Autodesk Inventor part; units mm, degrees
ref_plane "YZ Plane" through (0, 0, 0) normal (1, 0, 0) x (0, 1, 0)
ref_plane "XZ Plane" through (0, 0, 0) normal (0, 1, 0) x (-1, 0, 0)
ref_plane "XY Plane" through (0, 0, 0) normal (0, 0, 1) x (1, 0, 0)
sketch "Sketch1" plane through (0, 0, 0) normal (0, 0, 1) x (1, 0, 0)
  line L0 (-282.4704, -20.4341) -> (-282.4704, 20.4341)
  line L1 (-394.804, 0) -> (382.9893, 0) construction
  arc A0 (245.5307, -6.7859) -> (-282.4704, -20.4341) centre (0, -728.1449) ccw
  arc A1 (257.8072, 29.282) -> (-282.4704, 20.4341) centre (0, -728.1449) ccw
  line L2 (245.5307, -6.7859) -> (257.8072, 29.282)
  line L3 (257.8072, 29.282) -> (259.8533, 35.2933)
  line L4 (259.8533, 35.2933) -> (271.8759, 31.2011)
  line L5 (271.8759, 31.2011) -> (255.5072, -16.8895)
  line L6 (255.5072, -16.8895) -> (243.4846, -12.7973)
  line L7 (243.4846, -12.7973) -> (245.5307, -6.7859)
  line L8 (0, 237.1551) -> (0, -889.0282) construction
  line L9 (0, -728.1449) -> (-282.4704, 0) construction
  arc A2 (205.7125, -1.0346) -> (-280.1164, -26.3317) centre (0, -728.1449) ccw
  line L10 (-280.1164, -26.3317) -> (-282.4704, -20.4341)
  line L11 (243.4846, -12.7973) -> (245.5307, -6.7859)
  point P0 (0, 0)
  point P1 (205.7125, -1.0346)
  dimension "d65" = 762
  dimension "d67" = 50.8
  dimension "d68" = 38.1
  dimension "d69" = 12.7
  dimension "d76" = 40
  dimension "d97" = 800.1
  dimension "d98" = 6.35
extrude "Plate1" add sketch "Sketch1" along normal blind 4.7625 contours L0 A1 L2 A0
sketch "Sketch3" plane through (0, 0, 0) normal (0, 0, -1) x (-1, 0, 0)
  line L0 (269.2384, 95.4765) -> (282.4704, 20.4341)
  arc A0 (282.4704, 20.4341) -> (-257.8072, 29.282) centre (0, -728.1449) ccw
  arc A1 (282.4704, -20.4341) -> (-245.5307, -6.7859) centre (0, -728.1449) ccw construction
  line L1 (0, -900.8528) -> (0, 308.1027) construction
  line L2 (-366.2845, 0) -> (393.0567, 0) construction
  arc A2 (269.2384, 95.4765) -> (108.3857, 131.5609) centre (0, -728.1449) ccw
  arc A3 (108.3857, 131.5609) -> (104.0502, 97.172) centre (106.218, 114.3664) ccw
  arc A4 (203.8267, 78.347) -> (104.0502, 97.172) centre (0, -728.1449) ccw
  arc A5 (209.7927, 71.9287) -> (203.8267, 78.347) centre (201.8507, 70.5283) ccw
  line L3 (209.7927, 71.9287) -> (212.772, 55.032)
  arc A6 (202.7861, 45.8305) -> (212.772, 55.032) centre (204.8301, 53.6316) ccw
  point P0 (0, 0)
  point P1 (-2.2036, 71.9521)
  dimension "d70" = 80
  dimension "d88" = 165.1
  dimension "d91" = 76.2
  dimension "d92" = 101.6
  dimension "d93" = 8.0645
  dimension "d95" = 31.75
sheet face with bend "Face2" sketch "Sketch3" thickness 4.7625 toward (0, 0, 1) bend radius 4.7625
bend "Bend1"
sketch "Sketch5" plane through (0, 0, 0) normal (0, 0, -1) x (-1, 0, 0)
  arc A0 (282.4704, -20.4341) -> (-245.5307, -6.7859) centre (0, -728.1449) ccw construction
  spline S0 degree 3 poles (-4.2317, 35.5309) (-3.9947, 36.2065) (-3.5205, 37.5578) (-2.7876, 39.577) (-2.0409, 41.5912) (-1.5294, 42.9288) (-1.2737, 43.5976) knots 0 0 0 0 0.214807 0.429614 0.644422 0.859229 0.859229 0.859229 0.859229
  spline S1 degree 3 poles (4.2317, 35.5309) (3.9947, 36.2065) (3.5205, 37.5578) (2.7876, 39.577) (2.0409, 41.5912) (1.5294, 42.9288) (1.2737, 43.5976) knots 0 0 0 0 0.214807 0.429614 0.644422 0.859229 0.859229 0.859229 0.859229
  circle A1 centre (0, -728.1449) radius 763.6875
  arc A2 (1.2737, 43.5976) -> (-1.2737, 43.5976) centre (0, -728.1449) ccw
  point P0 (-3.5169, 37.5565)
  point P1 (-2.7853, 39.5762)
  point P2 (-2.0375, 41.5899)
  point P3 (3.5169, 37.5565)
  point P4 (2.7853, 39.5762)
  point P5 (2.0375, 41.5899)
extrude "Extrusion1" [suppressed]
pattern_circular "Circular Pattern1" [suppressed]
sketch "Sketch4" plane through (0, 0, 0) normal (0, 0, -1) x (-1, 0, 0)
  line L0 (282.4704, 20.4341) -> (269.2384, 95.4765) construction
  circle A0 centre (198.5568, 63.04) radius 25.4 construction
  line L1 (177.7503, 77.6089) -> (213.1256, 83.8465) construction
  line L2 (213.1256, 83.8465) -> (183.9879, 42.2336) construction
  line L3 (183.9879, 42.2336) -> (219.3632, 48.4712) construction
  line L4 (173.5426, 58.6294) -> (223.5709, 67.4507) construction
  line L5 (282.4704, 20.4341) -> (269.2384, 95.4765) construction
  line L6 (262.3523, 61.393) -> (265.6603, 42.6324) construction
  line L7 (0, -43.6162) -> (0, 118.6586) construction
  point P0 (0, 0)
  point P1 (257.9416, 86.4071)
  point P2 (272.2763, 5.1112)
  dimension "d31" = 25.4
  dimension "d33" = 12.7
  dimension "d34" = 12.7
  dimension "d42" = 50.8
  dimension "d43" = 45
  dimension "d51" = 5.2605
  dimension "d52" = 19.05
  dimension "d53" = 38.1
  dimension "d89" = 198.5568
  dimension "d90" = 63.04
hole "Hole2" at (-257.9416, 86.4071, 0) at (-262.3523, 61.393, 0) at (-177.7503, 77.6089, 0) at (-173.5426, 58.6294, 0) at (-183.9879, 42.2336, 0) at (-219.3632, 48.4712, 0) at (-223.5709, 67.4507, 0) at (-213.1256, 83.8465, 0) at (-272.2763, 5.1112, 0) at (-265.6603, 42.6324, 0) direction (0, 0, 1) diameter 5.105 end through all
feature "Corner Round4" [suppressed]
feature "Corner Round5" [suppressed]
fillet "Corner Round6" radius 6.35 1 edges at (-282.4704, -20.4341, 2.3813)
equation "\"d34\" = d32"
equation "\"d40\" = Thickness"
equation "\"d5\" = Thickness"
equation "\"d22\" = BendRadius"
equation "\"d23\" = BendReliefWidth"
equation "\"d25\" = MinimumRemnant"
equation "\"d24\" = BendReliefDepth"
equation "\"d26\" = TransitionRadius"
equation "\"BendRadius\" = Thickness"
equation "\"BendReliefWidth\" = Thickness"
equation "\"BendReliefDepth\" = 0.5 * Thickness"
equation "\"CornerReliefSize\" = 4 * Thickness"
equation "\"MinimumRemnant\" = 2 * Thickness"
equation "\"TransitionRadius\" = BendRadius"
equation "\"JacobiRadiusSize\" = BendRadius"
equation "\"GapSize\" = Thickness"
properties part number "RACK,INSIDE" material "Polycarbonate, PC 1000, Clear"
Could you check a few things on this model? Use its own coordinates, in mm. A direction names the side the tool comes from. Give positions to 0.01 mm unless a question says otherwise; leave off trailing zeros. Order: outer loops, then holes, each group sorted by start corner. A loop starts at its lowest first (then second) coordinate and runs counter-clockwise, first axis right, second up.
Q1. Suppose I cut it at A-A, the plane z = 1.2. Count the separate pieces of the cut face and the enclosed holes in it, and give its area (3 significant figures).
Q2. Suppose I cut it at B-B, the plane x = 87. Write out the boundary of the cut face in (y, z), and give its area (3 significant figures).
Q3. Suppose I cut it at C-C, the plane y = 118.5. Write out the boundary of the cut face in (x, z).
Q4. We'd pull the mould along Y, two halves only. Please class faces 1 (the flat face through (251.583, 10.996, 2.348)), 2 (the cylindrical face through (-210.211, 47.625, 2.348)), 3 (the cylindrical face through (-190.8, 117.1, 2.3)): +Y half, -Y half, draft (parallel to the pull), parting line (faces both ways), or undercut.
Q5. If I drill on line 1 along Y through (x, z) = (-257, 1.95); line 2 along Y through (x, z) = (213, 0.85); line 3 along Y through (x, z) = (-132, 3.1), over which ranges is the centre line in solid material (lowest first)?
Q6. For faces 4 (the flat face through (-275.76, 58.48, 2.35)), 5 (the cylindrical face through (25.46, 71.55, 2.35)), 6 (the cylindrical face through (-154.925, 89.151, 2.348)), which set-ups out of +Z, -Z, +X, -X, +Y, -Y let a thin tool reach every point of the face, with its end or its side?
Solution:
1. separate pieces: 1
1. enclosed holes: 8
1. area: 29,300 mm2
2. outline: (28.87, 0) - (67.21, 0) - (67.21, 4.76) - (28.87, 4.76) - close
2. area: 183 mm2
3. outline: (-184.48, 0) - (-89.39, 0) - (-89.39, 4.76) - (-184.48, 4.76) - close
4. face 1: -Y half
4. face 2: undercut
4. face 3: +Y half
5. line 1: y = -10.79 to 84.03, 88.78 to 99.38
5. line 2: y = 3.48 to 43.08
5. line 3: y = 22.34 to 60.99, 93.17 to 128.25
6. face 4: +Z, -Z, -X, +Y
6. face 5: +Z, -Z
6. face 6: +Z, -Z, +X
